Can you work these out from the model? Positions are in its coordinate system, mm. Face numbers are marked on the shaded views. Coordinates: 2 decimals unless noted, no trailing zeros. Loops run counter-clockwise (first coordinate to the right, second up) from the corner with the lowest first, then second, coordinate; pieces in that order, holes last. Notation, with made-up numbers: (52, 29.5) - (62, 29.5) arc R7 cw to (62, 39.5) - close; hole circle Ø9 at (-27, 68). An arc over 180 degrees is marked (long way). Put each result on its own line as item: value. Start each with the question number.
from build123d import *

# Parameters (mm, degrees)
F0_R     = 12.5
F1_DEPTH = 30
F2_DEPTH = 70
F3_R     = 1
F4_R     = 1
F5_R     = 0.5


with BuildPart() as f1:
    # F0 (on Front) → F1 (new body)
    with BuildSketch(Plane.XZ):
        with BuildLine():
            ThreePointArc((3.771303, -29.762011), (22.5071, -19.835081), (30, 0))
            ThreePointArc((30, 0), (22.98125, 19.283727), (5.209191, 29.544277))
            ThreePointArc((5.209191, 29.544277), (-29.991186, 0.72714), (3.771303, -29.762011))
        make_face()
        Circle(F0_R, mode=Mode.SUBTRACT)
        with BuildLine():
            ThreePointArc((5.209191, 29.544277), (22.98125, 19.283727), (30, 0))
            ThreePointArc((30, 0), (22.5071, -19.835081), (3.771303, -29.762011))
            Line((3.771303, -29.762011), (120.291015, -14.997177))
            ThreePointArc((120.291015, -14.997177), (105.020911, 0.791759), (121.870406, 14.882929))
            Line((121.870406, 14.882929), (5.209191, 29.544277))
        make_face()
        with BuildLine():
            ThreePointArc((135, 0), (131.248468, 9.923304), (121.870406, 14.882929))
            ThreePointArc((121.870406, 14.882929), (105.020911, 0.791759), (120.291015, -14.997177))
            ThreePointArc((120.291015, -14.997177), (130.708997, -10.503209), (135, 0))
        make_face()
        with Locations((120, 0)):
            Circle(F0_R, mode=Mode.SUBTRACT)
    extrude(amount=F1_DEPTH)

    # F0 (on Front) → F2 (join)
    with BuildSketch(Plane.XZ):
        with BuildLine():
            ThreePointArc((3.771303, -29.762011), (22.5071, -19.835081), (30, 0))
            ThreePointArc((30, 0), (22.98125, 19.283727), (5.209191, 29.544277))
            ThreePointArc((5.209191, 29.544277), (-29.991186, 0.72714), (3.771303, -29.762011))
        make_face()
        Circle(F0_R, mode=Mode.SUBTRACT)
    extrude(amount=F2_DEPTH)

    # F3
    f3_edges = [f1.edges().sort_by_distance(p)[0] for p in [
        (-3.771303, -70, 29.762011),
        (-12.5, -70, 0),
        (107.5, -30, 0),
    ]]
    fillet(f3_edges, radius=F3_R)

    # F4
    f4_edges = [f1.edges().sort_by_distance(p)[0] for p in [
        (-12.5, 0, 0),
    ]]
    fillet(f4_edges, radius=F4_R)

    # F5
    f5_edges = [f1.edges().sort_by_distance(p)[0] for p in [
        (107.5, 0, 0),
    ]]
    fillet(f5_edges, radius=F5_R)


solid = f1.part
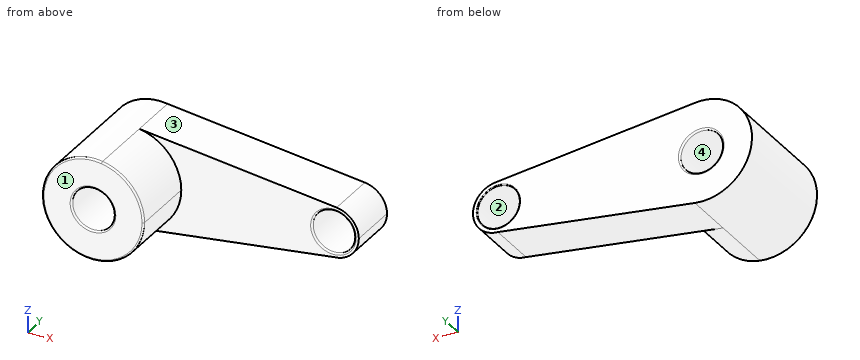
Q1. We'd pull the mould along X, two halves only. Please class the marked faces 1, 2, 3 and 4: released by +X, released by -X, zero draft, split by the parting line, or undercut.
Q2. I want a section at C-C on x = 40. List the corners of the cut face in (y, z) for me, and give its area (3 significant figures).
Q3. I want a section at A-A on y = -35. List the corners of the cut face in (x, z) for me, and give its area (3 significant figures).
Q4. I want a section at B-B on z = -9.5. Count the separate pieces of the cut face and the enclosed holes in it, and give its area (3 significant figures).
Q5. Please list where these lines run through material, in increasing order: line 1 along Z through (x, y) = (0, -33.5); line 2 along X through (y, z) = (-17.5, -4); line 3 along Y through (x, z) = (82.5, -1.5). Write a range as [from, to].
Q6. Will these pins go through, and if not, where does the flat tip stop? pin 1 (5 mm diameter, centred on y = -20.5, z = -13, fed in from -X); pin 2 (5 mm diameter, centred on y = -51.5, z = -4.5, fed in from +X); pin 3 (12 mm diameter, centred on y = -50.5, z = -13, fed in from +X).
Calculated:
1. face 1: zero draft
1. face 2: undercut
1. face 3: released by +X
1. face 4: undercut
2. outline: (-30, -25.17) - (0, -25.17) - (0, 25.17) - (-30, 25.17) - close
2. area: 1,510 mm2
3. outline: (3.77, -29.76) arc R30 ccw to (30, 0) arc R30 ccw (long way) to start; hole circle Ø25 at (0, 0)
3. area: 2,340 mm2
4. separate pieces: 3
4. enclosed holes: 0
4. area: 5,450 mm2
5. line 1: [-30, -12.5], [12.5, 30]
5. line 2: [-29.73, -11.84], [11.84, 108.16], [131.84, 134.46]
5. line 3: [-30, 0]
6. pin 1: x = -28.1
6. pin 2: x = 29.93
6. pin 3: x = 29.17
